Read the model definition and answer for the solid it produces. Units are mm, in the model's axes. A direction names the side the tool comes from. Coordinates: 2 decimals unless noted, no trailing zeros. Write each loop counter-clockwise with the first axis right and the second up, starting at its lowest first coordinate (ties: lowest second). Pieces come first, ordered by that corner, then holes.
1) Find the intervals of material crossed by line 1 (Y direction, x = 0, z = 3.75); line 2 (X direction, y = -52.5, z = 25); line 3 (X direction, y = -38, z = 1), in increasing order.
2) Determine the mould class of faces 4 (the face through (67.165, -38, 21)), 5 (the face through (-68.625, -38, 8)), 6 (the face through (70, -38, 31.101)) for opening direction X: +X half, -X half, draft (parallel to the pull), parting line (faces both ways), or undercut.
3) Which of the six approach directions +Z, -Z, +X, -X, +Y, -Y give full straight-line access (tool end or side, diameter ignored) to faces 1 (the face through (6.057, -36.193, 1.811)), 2 (the face through (2, -46, 9.638)), 3 (the face through (1, -38, -15.762))?
4) This flat-tipped pin is pushed along its axis until it touches: pin 1 Ø20.5 at (x, y) = (0, -38.1) entering from +Z. Where does it stop, or does it pass through?
5) The part is cut by section B-B (y = -51.5). Determine the outline of the cut face in (x, z), then the cut area to 3 significant figures.
6) The part is cut by section C-C (x = 0). Determine the outline of the cut face in (y, z), then the cut area to 3 significant figures.
7) The part is cut by section D-D (y = -38.1). Determine the outline of the cut face in (x, z), then the cut area to 3 significant figures.
8) The part is cut by section A-A (z = 24). Determine the outline of the cut face in (x, y).
from build123d import *

# Parameters (mm, degrees)
F1_DEPTH  = 76.2
F1_FACE_W = 12.7
F1_FACE_H = 76.2
F2_DEPTH  = 15.875
F3_R      = 6.35
F4_DEPTH  = 15.875


with BuildPart() as f1:
    # F0 (on Front) → F1 (new body)
    with BuildSketch(Plane.XZ):
        Polygon((-60.43807, 31.100702), (-68.62498, 31.100702), (-68.62498, -15.762298), (73.093257, -15.762298), (73.093257, 31.100702), (67.1648, 31.100702), (67.1648, 9.637702), (6.35, 9.637702), (6.35, -6.237298), (-6.35, -6.237298), (-6.35, 9.637702), (-60.43807, 9.637702), align=None)
    extrude(amount=F1_DEPTH)

    # F1_face (on face) → F2 (join)
    with BuildSketch(Plane(origin=(0, -38.1, -6.237298), x_dir=(1, 0, 0), z_dir=(0, 0, 1))):
        Rectangle(F1_FACE_W, F1_FACE_H)
    extrude(amount=F2_DEPTH)

    # F3 (on face) → F4 (cut)
    with BuildSketch(Plane.XY.offset(9.637702)):
        with Locations((0, -38.1)):
            Circle(F3_R)
    extrude(amount=-F4_DEPTH, mode=Mode.SUBTRACT)


solid = f1.part
Reported:
1. line 1: y = -76.2 to -44.45, -31.75 to 0
1. line 2: x = -68.62 to -60.44, 67.16 to 73.09
1. line 3: x = -68.62 to -6.35, 6.35 to 73.09
2. face 4: undercut
2. face 5: -X half
2. face 6: draft
3. face 1: +Z
3. face 2: +Z, +Y, -Y
3. face 3: -Z, +X, -X, +Y, -Y
4. pin 1: stops at z = 9.64
5. outline: (-68.62, -15.76) - (73.09, -15.76) - (73.09, 31.1) - (67.16, 31.1) - (67.16, 9.64) - (-60.44, 9.64) - (-60.44, 31.1) - (-68.62, 31.1) - close
5. area: 3,900 mm2
6. outline: (-76.2, -15.76) - (0, -15.76) - (0, 9.64) - (-31.75, 9.64) - (-31.75, -6.24) - (-44.45, -6.24) - (-44.45, 9.64) - (-76.2, 9.64) - close
6. area: 1,730 mm2
7. outline: (-68.62, -15.76) - (73.09, -15.76) - (73.09, 31.1) - (67.16, 31.1) - (67.16, 9.64) - (6.35, 9.64) - (6.35, -6.24) - (-6.35, -6.24) - (-6.35, 9.64) - (-60.44, 9.64) - (-60.44, 31.1) - (-68.62, 31.1) - close
7. area: 3,700 mm2
8. outline: (-68.62, -76.2) - (-60.44, -76.2) - (-60.44, 0) - (-68.62, 0) - close; (67.16, -76.2) - (73.09, -76.2) - (73.09, 0) - (67.16, 0) - close
